Can you work these out from the drawing? Everything is in mm from the part's minimum corner. A direction names the side the tool comes from. Round coordinates to 2 decimals unless told otherwise and drop trailing zeros. Write each loop counter-clockwise with the first axis right and the second up, starting at its lowest first coordinate (ties: lowest second). Pieces come first, ordered by that corner, then holes. Notation, with made-up numbers: M 66,3.5 L 120,3.5 A22 cw 120,13.5 Z; hole C -28,-11.5 d6. An arc over 180 degrees is marked long. Answer in a Markdown table with one row per item. Add a question column.
(1) Suppose I cut it at B-B, the plane y = 30. Write out the boundary of the cut face in (x, z).
(2) Suppose I cut it at A-A, the plane x = 26. Write out the boundary of the cut face in (y, z).
(3) If we mould it in two halves opening along Z, with no side actions, what happens to the marked faces 1, 2, 3 and 4? For each: released by +Z, released by -Z, zero draft, split by the parting line, or undercut.
(4) Suppose I cut it at D-D, the plane y = 49. Write out the boundary of the cut face in (x, z) (3 decimals), then the cut area to 3 significant figures.
(5) I'm going to push flat-ended pins straight in: pin 1 (3 mm diameter, centred on x = 28, z = 29.5, fed in from -Y); pin 2 (12 mm diameter, centred on x = 32.5, z = 43.5, fed in from -Y); pin 3 (1 mm diameter, centred on y = 23.5, z = 20.5, fed in from +X); pin 4 (18 mm diameter, centred on y = 30, z = 35, fed in from +X). Where does each tip first touch, or does it pass through?
(6) If I drill on probe 1 along Y at (x, z) = (29, 35); probe 2 along X at (y, z) = (27, 52); probe 3 along Z at (x, y) = (15, 38), over which ranges is the centre line in solid material (lowest first)?
(7) Suppose I cut it at C-C, the plane z = 41. Write out the boundary of the cut face in (x, y), then the cut area to 3 significant figures.
(8) For the marked faces 5, 6, 7 and 8, which set-ups out of +Z, -Z, +X, -X, +Y, -Y let a thin tool reach every point of the face, with its end or its side?
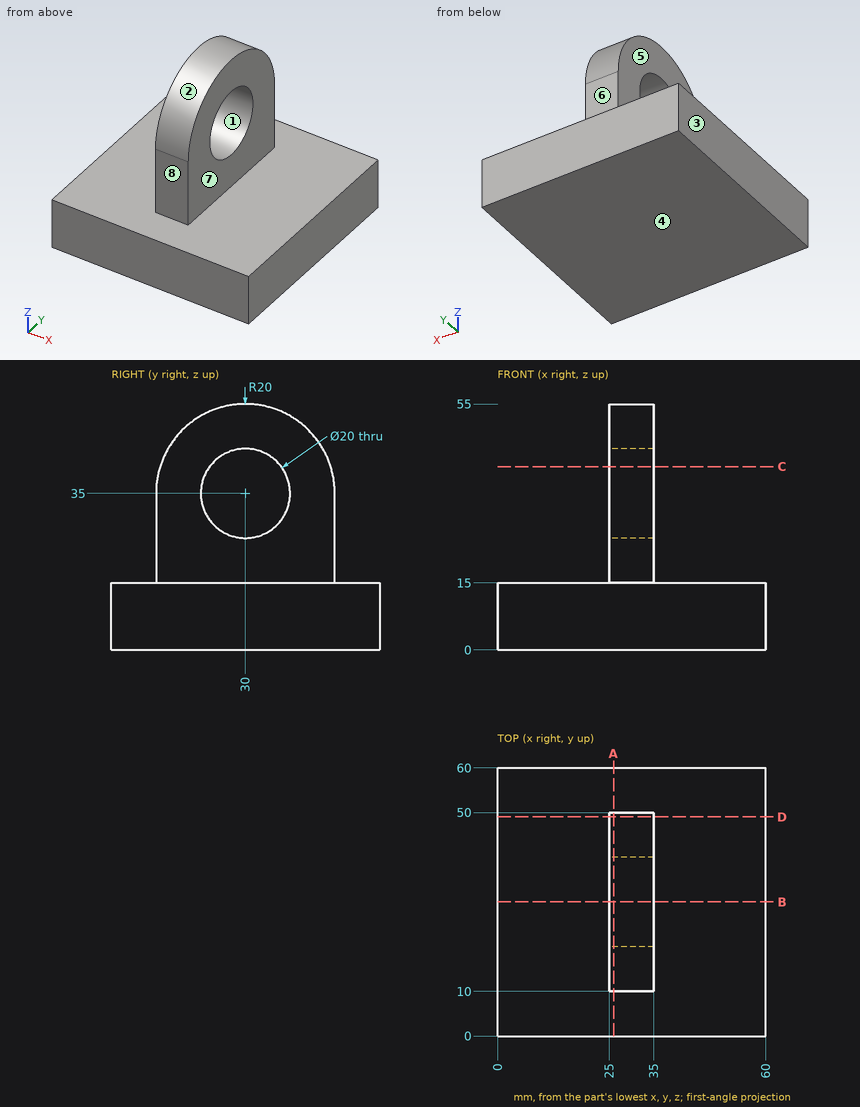
Calculated:
| question | item | result |
|---|---|---|
| 1 | outline | M 0,0 L 60,0 L 60,15 L 35,15 L 35,25 L 25,25 L 25,15 L 0,15 Z; M 25,45 L 35,45 L 35,55 L 25,55 Z |
| 2 | outline | M 0,0 L 60,0 L 60,15 L 50,15 L 50,35 A20 ccw 10,35 L 10,15 L 0,15 Z; hole C 30,35 d20 |
| 3 | face 1 | undercut |
| 3 | face 2 | released by +Z |
| 3 | face 3 | zero draft |
| 3 | face 4 | released by -Z |
| 4 | outline | M 0,0 L 60,0 L 60,15 L 35,15 L 35,41.245 L 25,41.245 L 25,15 L 0,15 Z |
| 4 | area | 1,160 mm² |
| 5 | pin 1 | y = 10 |
| 5 | pin 2 | y = 10.16 |
| 5 | pin 3 | x = 35 |
| 5 | pin 4 | through |
| 6 | probe 1 | 10 to 20, 40 to 50 |
| 6 | probe 2 | 25 to 35 |
| 6 | probe 3 | 0 to 15 |
| 7 | outline | M 25,10.92 L 35,10.92 L 35,22 L 25,22 Z; M 25,38 L 35,38 L 35,49.08 L 25,49.08 Z |
| 7 | area | 222 mm² |
| 8 | face 5 | +Z, -X, +Y, -Y |
| 8 | face 6 | +Z, +X, -X, +Y |
| 8 | face 7 | +Z, +X, +Y, -Y |
| 8 | face 8 | +Z, +X, -X, -Y |
